```python
from build123d import *

# Parameters (mm, degrees)
SKETCH1_R           = 2.014647572
BOSS_EXTRUDE1_DEPTH = 1.5
SKETCH2_R           = 6.338534982
SKETCH2_W           = 4.270612397
SKETCH2_H           = 5.923752679
BOSS_EXTRUDE2_DEPTH = 3


with BuildPart() as part:
    # Sketch1 → Boss-Extrude1 (new body)
    with BuildSketch(Plane.XY):
        Polygon((6.096678716, 18.525469925), (6.096678716, 41.025469925), (14.504757975, 41.025469925), (14.504757975, 55.525469925), (84.004757975, 55.525469925), (84.004757975, 97.525469925), (99.504757975, 97.525469925), (99.504757975, 90.525469925), (92.096678716, 90.525469925), (92.096678716, 38.525469925), (106.096678716, 38.525469925), (106.096678716, 18.525469925), (70.532495119, 18.525469925), align=None)
        with Locations((96.096678716, 35.525469925)):
            Circle(SKETCH1_R, mode=Mode.SUBTRACT)
        with Locations((96.096678716, 93.874977547)):
            Circle(SKETCH1_R, mode=Mode.SUBTRACT)
        with Locations((10.096678716, 35.525469925)):
            Circle(SKETCH1_R, mode=Mode.SUBTRACT)
    extrude(amount=BOSS_EXTRUDE1_DEPTH)

    # Sketch2 → Boss-Extrude2 (add)
    with BuildSketch(Plane.XY.offset(1.5)):
        with Locations(Location((23.665238751, 23.02282619, 0), (0, 0, 225.19637393))):
            Circle(SKETCH2_R)
        with Locations((44.536134816, 23.367230416)):
            Rectangle(SKETCH2_W, SKETCH2_H)
    extrude(amount=BOSS_EXTRUDE2_DEPTH)


solid = part.part
```
Work out the finished part from the listing and answer in its coordinate system (mm). A direction names the side the tool comes from. Round coordinates to 2 decimals unless told otherwise and drop trailing zeros. Write each loop counter-clockwise with the first axis right and the second up, starting at its lowest first coordinate (ties: lowest second). Pieces come first, ordered by that corner, then holes.
1) Consider probe 1 along Z at (x, y) = (64, 38.5); probe 2 along X at (y, z) = (91, 0.55); probe 3 along Y at (x, z) = (97, 0.5). Determine where each line is inside the solid, lowest interval first.
2) Flat-ended cylindrical pins translate along their axes: P1, Ø1, axis at x = 55.5, z = 0.5, coming from the +Y side; P2, Ø1.6, axis at x = 69.5, z = 1, coming from the -Y side; P3, Ø1.5, axis at x = 44, z = 2.5, coming from the -Y side. Find the tip coordinate at first contact, or state that the pin passes through.
3) A cutting plane is placed at B-B on x = 27. Determine the outline of the cut face in (y, z).
4) A cutting plane is placed at C-C on y = 81. Determine the outline of the cut face in (x, z), and give its area (3 significant figures).
5) Which of the six approach directions +Z, -Z, +X, -X, +Y, -Y give full straight-line access (tool end or side, diameter ignored) to faces 4 (the face through (45, 26.329, 3)), 5 (the face through (42.401, 23, 3)), 6 (the face through (45, 20.405, 3))?
6) A cutting plane is placed at D-D on x = 44.5. Determine the outline of the cut face in (y, z), and give its area (3 significant figures).
7) Determine the mould class of faces 1 (the face through (95.834, 37.523, 0.74)), 2 (the face through (20.243, 28.358, 2.979)), 3 (the face through (46.671, 23, 3)) for opening direction Y: pulls with the +Y half, pulls with the -Y half, needs draft (parallel to the pull), parting line crosses it, or undercut.
8) A cutting plane is placed at A-A on z = 3.7. Determine the outline of the cut face in (x, y), and give its area (3 significant figures).
Entries:
1. probe 1: z = 0 to 1.5
1. probe 2: x = 84 to 99.5
1. probe 3: y = 18.53 to 33.72, 37.33 to 38.53, 90.53 to 92.07, 95.68 to 97.53
2. P1: stops at y = 55.53
2. P2: stops at y = 18.53
2. P3: stops at y = 20.41
3. outline: (17.63, 1.5) - (18.53, 1.5) - (18.53, 0) - (55.53, 0) - (55.53, 1.5) - (28.41, 1.5) - (28.41, 4.5) - (17.63, 4.5) - close
4. outline: (84, 0) - (92.1, 0) - (92.1, 1.5) - (84, 1.5) - close
4. area: 12.1 mm2
5. face 4: +Z, +X, +Y
5. face 5: +Z, +Y, -Y
5. face 6: +Z, +X, -Y
6. outline: (18.53, 0) - (55.53, 0) - (55.53, 1.5) - (26.33, 1.5) - (26.33, 4.5) - (20.41, 4.5) - (20.41, 1.5) - (18.53, 1.5) - close
6. area: 73.3 mm2
7. face 1: undercut
7. face 2: parting line crosses it
7. face 3: needs draft
8. outline: circle Ø12.68 at (23.67, 23.02); (42.4, 20.41) - (46.67, 20.41) - (46.67, 26.33) - (42.4, 26.33) - close
8. area: 152 mm2
